Here's how the part is built. I have some questions about the finished solid (model axes, mm). Give positions to 0.01 mm unless a question says otherwise; leave off trailing zeros. Loops run counter-clockwise (first coordinate to the right, second up) from the corner with the lowest first, then second, coordinate; pieces in that order, holes last. Notation, with made-up numbers: (26.5, -39.5) - (72.5, -39.5) arc R27 cw to (72.5, -17.5) - close; hole circle Ø1 at (-36.75, -27). An arc over 180 degrees is marked (long way). Use one line per item in the form item = value.
Autodesk Inventor part; units mm, degrees
ref_plane "rr_XY" through (-1, 0, 0) normal (1, 0, 0) x (0, 0, -1)
ref_plane "rr_YZ" through (-1, 0, 0) normal (0, 0, -1) x (0, 1, 0)
ref_plane "rr_ZX" through (-1, 0, 0) normal (0, 1, 0) x (1, 0, 0)
sketch "Sketch_3" plane through (0, 0, 0) normal (1, 0, 0) x (0, 1, 0)
  arc A0 (-26.7266, -11.2556) -> (-26.7266, 11.2556) centre (0, 0) ccw
  arc A1 (-26.7266, 11.2556) -> (-25.1712, 7.9) centre (-24.4226, 10.2853) ccw
  line L0 (-25.1712, 7.9) -> (-24.3719, 7.6491)
  arc A2 (-24.3719, 7.6491) -> (-20.6636, 12.5054) centre (-23.3987, 10.75) ccw
  arc A3 (-20.397, 16.3747) -> (-20.6636, 12.5054) centre (-17.9284, 14.2608) ccw
  arc A4 (-20.397, -16.3747) -> (-20.397, 16.3747) centre (-1.275, 0) ccw
  arc A5 (-20.6636, -12.5054) -> (-20.397, -16.3747) centre (-17.9284, -14.2608) ccw
  arc A6 (-20.6636, -12.5054) -> (-24.3719, -7.6491) centre (-23.3987, -10.75) ccw
  line L1 (-24.3719, -7.6491) -> (-25.1712, -7.9)
  arc A7 (-25.1712, -7.9) -> (-26.7266, -11.2556) centre (-24.4226, -10.2853) ccw
  circle A8 centre (-23.3987, -10.75) radius 1.25
  circle A9 centre (-23.3987, 10.75) radius 1.25
extrude "Extrusion1" add sketch "Sketch_3" along normal mid plane 2
ref_plane "rr_XY" through (-1, 0, 0) normal (1, 0, 0) x (0, 0, -1)
ref_plane "rr_YZ" through (-1, 0, 0) normal (0, 0, -1) x (0, 1, 0)
ref_plane "rr_ZX" through (-1, 0, 0) normal (0, 1, 0) x (1, 0, 0)
properties part number "RRING-C-INT-S-55"
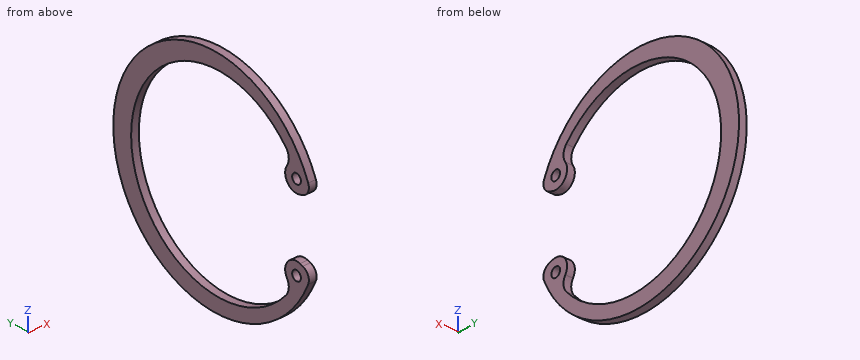
(1) For P1, Ø3, axis at y = 22.5, z = -22.5, coming from the -X side; P2, Ø3, axis at y = -23.4, z = 10.75, coming from the +X side, each with a flat end and sliding along its axis, tell me the tip position at first contact or that it passes through.
Geometry says:
P1 = through
P2 = 1
(2) If we section it at D-D (z = 0): List the corners of the cut face in (x, y) for me, plus the area to 3 significant figures.
Geometry says:
outline = (-1, 23.9) - (1, 23.9) - (1, 29) - (-1, 29) - close
area = 10.2 mm²
(3) If we section it at C-C (x = 0.2): List the corners of the cut face in (y, z) for me (3 decimals).
Geometry says:
outline = (-26.727, -11.256) arc R29 ccw (long way) to (-26.727, 11.256) arc R2.5 ccw to (-25.171, 7.9) - (-24.372, 7.649) arc R3.25 ccw to (-20.664, 12.505) arc R3.25 cw to (-20.397, 16.375) arc R25.175 cw (long way) to (-20.397, -16.375) arc R3.25 cw to (-20.664, -12.505) arc R3.25 ccw to (-24.372, -7.649) - (-25.171, -7.9) arc R2.5 ccw to start; hole circle Ø2.5 at (-23.399, -10.75); hole circle Ø2.5 at (-23.399, 10.75)
(4) If we section it at A-A (z = -15.5): List the corners of the cut face in (x, y) for me, plus the area to 3 significant figures.
Geometry says:
outline = (-1, -24.51) - (1, -24.51) - (1, -20.93) - (-1, -20.93) - close; (-1, 18.56) - (1, 18.56) - (1, 24.51) - (-1, 24.51) - close
area = 19.0 mm²
(5) If I drill on probe 1 along Z at (x, y) = (-0.45, 13); probe 2 along Y at (x, z) = (0.35, 0); probe 3 along Z at (x, y) = (0.2, 19), over which ranges is the centre line in solid material (lowest first)?
Geometry says:
probe_1 = -25.92 to -20.74, 20.74 to 25.92
probe_2 = 23.9 to 29
probe_3 = -21.91 to -14.92, 14.92 to 21.91
(6) If we section it at B-B (y = -17.5): List the corners of the cut face in (x, z) for me.
Geometry says:
outline = (-1, -23.12) - (1, -23.12) - (1, -19.25) - (-1, -19.25) - close; (-1, 19.25) - (1, 19.25) - (1, 23.12) - (-1, 23.12) - close
